from build123d import *

# Parameters (mm, degrees)
CROQUIS1_W              = 47
CROQUIS1_H              = 40.5
SALIENTE_EXTRUIR1_DEPTH = 25
CROQUIS2_W              = 10.933851529
CROQUIS2_H              = 3
SALIENTE_EXTRUIR2_DEPTH = 25
CROQUIS3_W              = 38.25
CROQUIS3_H              = 31.25
CORTAR_EXTRUIR1_DEPTH   = 22.5
CROQUIS6_R              = 15.25
CORTAR_EXTRUIR2_DEPTH   = 10
SALIENTE_EXTRUIR5_START = 4.75
CROQUIS7_W              = 47
CROQUIS7_H              = 40.5
CROQUIS7_R              = 15.25
SALIENTE_EXTRUIR5_DEPTH = 4.75
CROQUIS8_W              = 25
CROQUIS8_H              = 4
SALIENTE_EXTRUIR6_DEPTH = 3
CROQUIS9_R              = 1
SALIENTE_EXTRUIR7_DEPTH = 10


with BuildPart() as part:
    # Croquis1 → Saliente-Extruir1 (new body)
    with BuildSketch(Plane.XY.offset(25)):
        with Locations((-22.24307249, 34.18630066)):
            Rectangle(CROQUIS1_W, CROQUIS1_H)
    extrude(amount=-SALIENTE_EXTRUIR1_DEPTH)

    # Croquis2 → Saliente-Extruir2 (add)
    with BuildSketch(Plane.ZY.offset(45.74307249)):
        with Locations((19.533074236, 32.04630066)):
            Rectangle(CROQUIS2_W, CROQUIS2_H)
    extrude(amount=SALIENTE_EXTRUIR2_DEPTH)

    # Croquis3 → Cortar-Extruir1 (cut)
    with BuildSketch(Plane.XY.offset(25)):
        with Locations((-22.86807249, 34.56130066)):
            Rectangle(CROQUIS3_W, CROQUIS3_H)
    extrude(amount=-CORTAR_EXTRUIR1_DEPTH, mode=Mode.SUBTRACT)

    # Croquis6 → Cortar-Extruir2 (cut)
    with BuildSketch(Plane(origin=(0, 0, 0), x_dir=(-1, 0, 0), z_dir=(0, 0, -1))):
        with Locations((22.24307249, 34.18630066)):
            Circle(CROQUIS6_R)
    extrude(amount=-CORTAR_EXTRUIR2_DEPTH, mode=Mode.SUBTRACT)

    # Croquis7 → Saliente-Extruir5 (add)
    with BuildSketch(Plane(origin=(0, 0, 0), x_dir=(-1, 0, 0), z_dir=(0, 0, -1)).offset(SALIENTE_EXTRUIR5_START)):
        with Locations((22.24307249, 34.18630066)):
            Rectangle(CROQUIS7_W, CROQUIS7_H)
        with Locations((22.24307249, 34.18630066)):
            Circle(CROQUIS7_R, mode=Mode.SUBTRACT)
    extrude(amount=-SALIENTE_EXTRUIR5_DEPTH)

    # Croquis8 → Saliente-Extruir6 (add)
    with BuildSketch(Plane(origin=(0, 33.54630066, 0), x_dir=(1, 0, 0), z_dir=(0, 1, 0))):
        with Locations((-58.24307249, -27)):
            Rectangle(CROQUIS8_W, CROQUIS8_H)
    extrude(amount=-SALIENTE_EXTRUIR6_DEPTH)

    # Croquis9 → Saliente-Extruir7 (add)
    with BuildSketch(Plane(origin=(0, 33.54630066, 0), x_dir=(1, 0, 0), z_dir=(0, 1, 0))):
        with Locations(Location((-61.24307249, -26.590447053, 0), (0, 0, 90))):
            Circle(CROQUIS9_R)
        with Locations(Location((-51.74307249, -26.590447053, 0), (0, 0, 90))):
            Circle(CROQUIS9_R)
    extrude(amount=SALIENTE_EXTRUIR7_DEPTH)


solid = part.part
The model under review builds one solid part; all positions refer to its coordinate system, in mm. A direction names the side the tool comes from. Give positions to 0.01 mm unless a question says otherwise; leave off trailing zeros. Order: outer loops, then holes, each group sorted by start corner. A loop starts at its lowest first (then second) coordinate and runs counter-clockwise, first axis right, second up. Notation, with made-up numbers: M 74.5,-19 L 104.5,-19 A22 cw 104.5,18 Z; hole C 42.25,-24.75 d6. An arc over 180 degrees is marked long. Use one line per item in the form item = value. Start each with the question number.
Item 1: We need section B-B on y = 29.5. Give the boundary of the cut face in (x, z).
Item 2: To check wall thickness, follow line 1 along X through (y, z) = (49.5, 24); line 2 along Y through (x, z) = (-5, 7.5); line 3 along Z through (x, y) = (-4.5, 33.5). State the ranges of each line that lie inside material, in increasing order. Write a range as from..to.
Item 3: The part is to be moulded in two halves that separate along X. For faces 5 (the flat face through (-22, 54.436, 10)), 6 (the flat face through (-70.743, 32, 22)), 7 (the flat face through (-23, 50.186, 14)), say which applies: pulls with the +X half, pulls with the -X half, needs draft (parallel to the pull), parting line crosses it, or undercut.
Item 4: We need section D-D on x = -6. Give the boundary of the cut face in (y, z).
Item 5: We need section A-A on z = 23. Give the boundary of the cut face in (x, y), plus the area to 3 significant figures.
Item 6: We need section C-C on x = -26.5. Give the boundary of the cut face in (y, z), plus the area to 3 significant figures.
Item 7: Insertion check: pin 1 Ø0.9 at (x, y) = (-62.5, 31.5) entering from -Z; pin 2 Ø12 at (x, z) = (-52, 22) entering from -Y; pin 3 Ø2 at (y, z) = (33.5, 10.5) entering from -X; pin 4 Ø5 at (x, y) = (-16, 45) entering from -Z. Each pin has a flat end and moves straight along its axis. Give the tip position at first contact, or say it passes through.
Item 8: For faces 1 (the flat face through (-23, 18.936, 14)), 2 (the flat face through (-58, 32, 14.066)), 3 (the flat face through (-45.743, 32, 27)), 4 (the cylindrical face through (-62.086, 38.476, 26.053)), list the 3-axis set-ups (+Z, -Z, +X, -X, +Y, -Y) from which the entire face can be reached by the end or side of a thin tool; tool diameter is ignored.
Completed:
q1.outline = M -45.74,-4.75 L -36.76,-4.75 L -36.76,2.5 L -41.99,2.5 L -41.99,25 L -45.74,25 Z; M -7.73,-4.75 L 1.26,-4.75 L 1.26,25 L -3.74,25 L -3.74,2.5 L -7.73,2.5 Z
q2.line_1 = -45.74..-41.99, -3.74..1.26
q2.line_2 = 13.94..18.94, 50.19..54.44
q2.line_3 = -4.75..2.5
q3.face_5 = needs draft
q3.face_6 = pulls with the -X half
q3.face_7 = undercut
q4.outline = M 13.94,-4.75 L 54.44,-4.75 L 54.44,25 L 50.19,25 L 50.19,2.5 L 18.94,2.5 L 18.94,25 L 13.94,25 Z
q5.outline = M -70.74,30.55 L -45.74,30.55 L -45.74,13.94 L 1.26,13.94 L 1.26,54.44 L -45.74,54.44 L -45.74,33.55 L -70.74,33.55 Z; hole M -41.99,18.94 L -3.74,18.94 L -3.74,50.19 L -41.99,50.19 Z
q5.area = 783 mm²
q6.outline = M 13.94,-4.75 L 19.54,-4.75 L 19.54,2.5 L 18.94,2.5 L 18.94,25 L 13.94,25 Z; M 48.83,-4.75 L 54.44,-4.75 L 54.44,25 L 50.19,25 L 50.19,2.5 L 48.83,2.5 Z
q6.area = 289 mm²
q7.pin_1 = 14.07
q7.pin_2 = 30.55
q7.pin_3 = -45.74
q7.pin_4 = through
q8.face_1 = +Z
q8.face_2 = -Z, -X, +Y, -Y
q8.face_3 = +Z, +X, +Y, -Y
q8.face_4 = +Y
